Check sheet for the modelled part. Datum: model origin and axes. Units: mm. Face numbers are marked on the shaded views. A direction names the side the tool comes from. Coordinates: 2 decimals unless noted, no trailing zeros. Order: outer loops, then holes, each group sorted by start corner. A loop starts at its lowest first (then second) coordinate and runs counter-clockwise, first axis right, second up.
1. Gauge pin test, flat ends, axial feed: pin 1 Ø5.5 at (x, y) = (5, 84.6) entering from +Z; pin 2 Ø14 at (x, z) = (12.5, -19) entering from +Y; pin 3 Ø11 at (x, z) = (14, -14) entering from +Y. Record the tip position at first contact, or that the pin passes through.
2. Cross-section at B-B (z = -25). Enter the section's corners in (x, y).
3. Draft check along X on the marked faces 3, 4 and 5. Enter one of: released by +X, released by -X, zero draft, split by the parting line, or undercut.
4. Cross-section at A-A (x = 14). Enter the section's corners in (y, z), then the cut area to 3 significant figures.
5. Cross-section at C-C (z = -3.5). Enter the section's corners in (x, y).
6. Set-up check for the marked faces 1 and 2: record each of +Z, -Z, +X, -X, +Y, -Y from which the full face is reachable in a straight line by a thin tool's end or side.
7. Thickness scan on line 1 (X direction, y = 2.3, z = -14); line 2 (X direction, y = 6.2, z = -30.5); line 3 (X direction, y = 84, z = -30). Record the ranges inside material, lowest first.
8. Cross-section at D-D (y = 42). Enter the section's corners in (x, z).
```python
from build123d import *

# Parameters (mm, degrees)
SKETCH1_W           = 28
SKETCH1_H           = 28
SKETCH1_R           = 3
SKETCH1_R_2         = 1.7
BOSS_EXTRUDE1_DEPTH = 4.5
SKETCH2_W           = 28
SKETCH2_H           = 94.6
BOSS_EXTRUDE2_DEPTH = 4.545037206
SKETCH3_R           = 1.7
CUT_EXTRUDE1_DEPTH  = 103.553205703
SKETCH5_R           = 9
CUT_EXTRUDE2_DEPTH  = 2


with BuildPart() as part:
    # Sketch1 → Boss-Extrude1 (new body)
    with BuildSketch(Plane(origin=(0, 0, 0), x_dir=(1, 0, 0), z_dir=(0, 1, 0))):
        with Locations((14, 14)):
            Rectangle(SKETCH1_W, SKETCH1_H)
        with Locations(Location((14, 14, 0), (0, 0, 270))):
            Circle(SKETCH1_R, mode=Mode.SUBTRACT)
        with Locations(Location((14, 25, 0), (0, 0, 270))):
            Circle(SKETCH1_R_2, mode=Mode.SUBTRACT)
        with Locations(Location((25, 14, 0), (0, 0, 270))):
            Circle(SKETCH1_R_2, mode=Mode.SUBTRACT)
        with Locations(Location((14, 3, 0), (0, 0, 270))):
            Circle(SKETCH1_R_2, mode=Mode.SUBTRACT)
        with Locations(Location((3, 14, 0), (0, 0, 270))):
            Circle(SKETCH1_R_2, mode=Mode.SUBTRACT)
    extrude(amount=BOSS_EXTRUDE1_DEPTH)

    # Sketch2 → Boss-Extrude2 (add)
    with BuildSketch(Plane(origin=(0, 0, -28), x_dir=(-1, 0, 0), z_dir=(0, 0, -1))):
        with Locations((-14, 47.3)):
            Rectangle(SKETCH2_W, SKETCH2_H)
    extrude(amount=BOSS_EXTRUDE2_DEPTH)

    # Sketch3 → Cut-Extrude1 (cut, through all)
    with BuildSketch(Plane.XY.offset(-28)):
        with Locations((5, 6.2)):
            Circle(SKETCH3_R)
        with Locations((5, 84.6)):
            Circle(SKETCH3_R)
        with Locations(Location((23, 6.2, 0), (0, 0, 270))):
            Circle(SKETCH3_R)
        with Locations(Location((23, 84.6, 0), (0, 0, 180))):
            Circle(SKETCH3_R)
    extrude(amount=-CUT_EXTRUDE1_DEPTH, mode=Mode.SUBTRACT)

    # Sketch5 → Cut-Extrude2 (cut)
    with BuildSketch(Plane(origin=(0, 4.5, 0), x_dir=(1, 0, 0), z_dir=(0, 1, 0))):
        with Locations(Location((14, 14, 0), (0, 0, 270))):
            Circle(SKETCH5_R)
    extrude(amount=-CUT_EXTRUDE2_DEPTH, mode=Mode.SUBTRACT)


solid = part.part
```
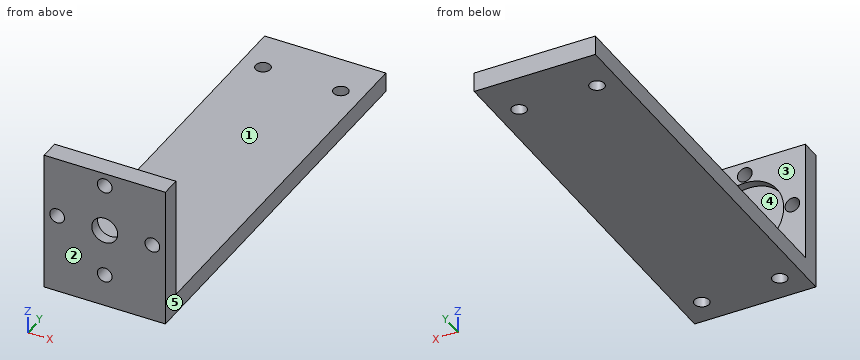
Data:
1. pin 1: stops at z = -28
1. pin 2: stops at y = 4.5
1. pin 3: stops at y = 2.5
2. outline: (0, 0) - (12.3, 0) - (12.3, 4.5) - (0, 4.5) - close; (15.7, 0) - (28, 0) - (28, 4.5) - (15.7, 4.5) - close
3. face 3: zero draft
3. face 4: undercut
3. face 5: released by +X
4. outline: (0, -32.55) - (94.6, -32.55) - (94.6, -28) - (4.5, -28) - (4.5, -26.7) - (0, -26.7) - close; (0, -23.3) - (4.5, -23.3) - (4.5, -23) - (2.5, -23) - (2.5, -17) - (0, -17) - close; (0, -11) - (2.5, -11) - (2.5, -5) - (4.5, -5) - (4.5, -4.7) - (0, -4.7) - close; (0, -1.3) - (4.5, -1.3) - (4.5, 0) - (0, 0) - close
4. area: 474 mm2
5. outline: (0, 0) - (12.38, 0) - (12.38, 4.5) - (0, 4.5) - close; (15.62, 0) - (28, 0) - (28, 4.5) - (15.62, 4.5) - close
6. face 1: +Z, +X, -X, +Y
6. face 2: +Z, -Z, +X, -X, -Y
7. line 1: x = 0 to 1.3, 4.7 to 11, 17 to 23.3, 26.7 to 28
7. line 2: x = 0 to 3.3, 6.7 to 21.3, 24.7 to 28
7. line 3: x = 0 to 3.41, 6.59 to 21.41, 24.59 to 28
8. outline: (0, -32.55) - (28, -32.55) - (28, -28) - (0, -28) - close
